Geometry: see drawing. Coordinates: mm, zero at the bounding-box minimum. A direction names the side the tool comes from. Coordinates: 2 decimals unless noted, no trailing zeros. Order: outer loops, then holes, each group sorted by start corner. A loop starts at its lowest first (then second) coordinate and runs counter-clockwise, first axis right, second up.
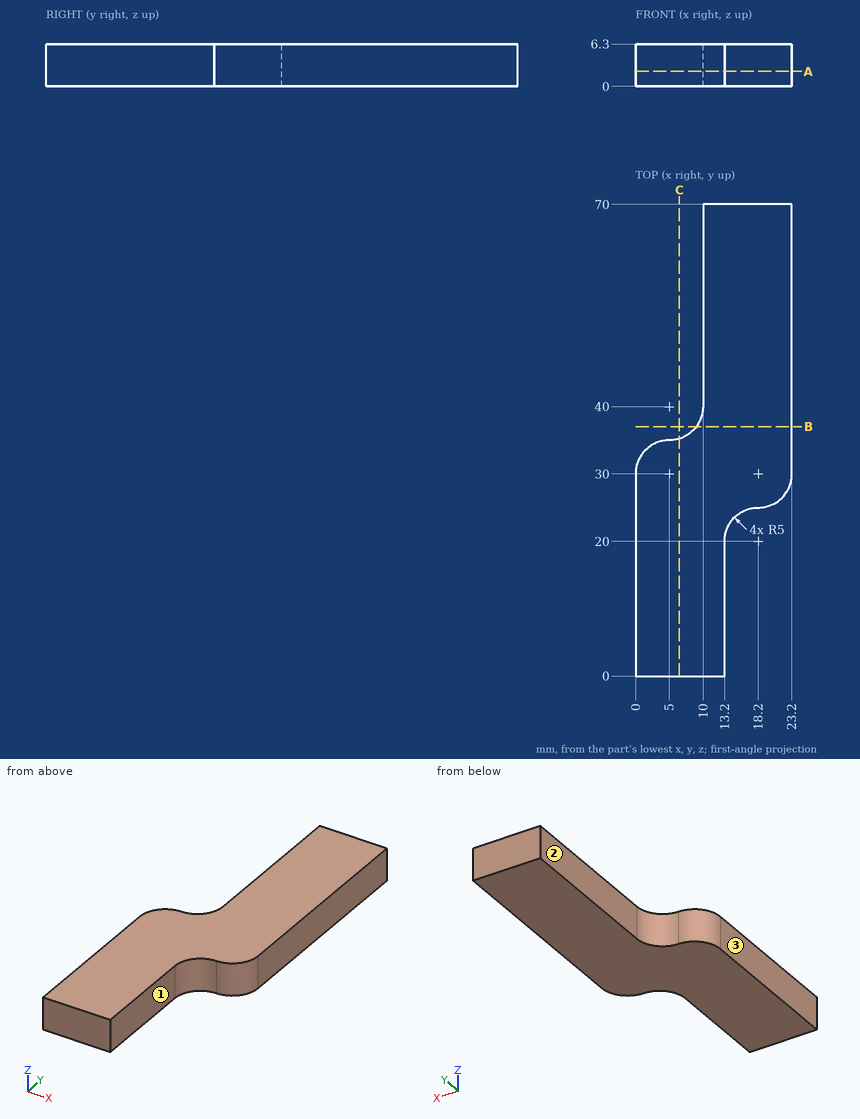
Q1. Set-up query: the marked faces 1, 2 and 3. Return all of +Z, -Z, +X, -X, +Y, -Y with unobstructed straight access to the full face (end or side cutting, diameter ignored); none if empty.
Solutions:
face 1: +Z, -Z, +X, -Y
face 2: +Z, -Z, -X, +Y
face 3: +Z, -Z, -X, +Y, -Y
Q2. Section query C-C on x = 6.5. Output: boundary loops of the cut face in (y, z), plus the area to 3 significant figures.
Solutions:
outline: (0, 0) - (35.23, 0) - (35.23, 6.3) - (0, 6.3) - close
area: 222 mm2
Q3. Section query B-B on y = 37. Output: boundary loops of the cut face in (x, z), plus the area to 3 significant figures.
Solutions:
outline: (9, 0) - (23.2, 0) - (23.2, 6.3) - (9, 6.3) - close
area: 89.5 mm2
Q4. Pin query (flat end, axial travel): P1, Ø1.5, axis at y = 44, z = 1.5, coming from the -X side; P2, Ø10, axis at x = 3.5, y = 41.5, coming from the +Z side. Return the tip coordinate at first contact, or that it passes through.
Solutions:
P1: stops at x = 10
P2: passes through
Q5. Section query A-A on z = 2.25. Output: boundary loops of the cut face in (x, y).
Solutions:
outline: (0, 0) - (13.2, 0) - (13.2, 20) arc R5 cw to (18.2, 25) arc R5 ccw to (23.2, 30) - (23.2, 70) - (10, 70) - (10, 40) arc R5 cw to (5, 35) arc R5 ccw to (0, 30) - close
Q6. Material intervals for line 1 along X through (y, z) = (59.5, 2.75); line 2 along X through (y, z) = (5, 6); line 3 along Y through (x, z) = (17.5, 3.5), sorted ascending.
Solutions:
line 1: x = 10 to 23.2
line 2: x = 0 to 13.2
line 3: y = 24.95 to 70
